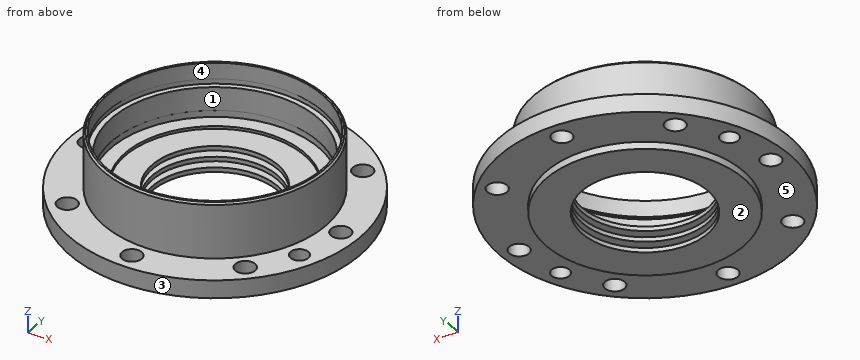
```python
from build123d import *

# Parameters (mm, degrees)
SKETCH_1_R               = 55
EXTRUDE_1_DEPTH          = 4
SKETCH_2_R               = 81
EXTRUDE_2_DEPTH          = 10
EXTRUDE_START            = 14
SKETCH_3_R               = 62
EXTRUDE_3_DEPTH          = 31
HOLE_WIZARD_1_D          = 11
PATTERN_CIRCULAR_1_COUNT = 8
HOLE_START               = 4
HOLE_WIZARD_2_OUTLINE_R  = 5
HOLE_WIZARD_2_DEPTH      = 10
CHAMFER_1_SIZE           = 1


# Read off the part's stored shape, not the designer's step: 孔2
with BuildPart() as part:
    # 草图1 → 凸台-拉伸1 (new body)
    with BuildSketch(Plane.XY):
        Circle(SKETCH_1_R)
    extrude(amount=EXTRUDE_1_DEPTH)

    # 草图2 → 凸台-拉伸2 (add)
    with BuildSketch(Plane.XY.offset(4)):
        Circle(SKETCH_2_R)
    extrude(amount=EXTRUDE_2_DEPTH)

    # 草图3 → 凸台-拉伸3 (add)
    with BuildSketch(Plane.XY.offset(EXTRUDE_START)):
        Circle(SKETCH_3_R)
    extrude(amount=EXTRUDE_3_DEPTH)

    # 草图4 → 切除-旋转1 (revolve, cut)
    with BuildSketch(Plane(origin=(0, 0, 0), x_dir=(0, 0, -1), z_dir=(1, 0, 0)), mode=Mode.PRIVATE) as cut_revolve_1_sk:
        Polygon((-45, 0), (-45, -60), (-36, -60), (-36, -60.5), (-33, -60.5), (-33, -57.5), (-20, -57.5), (-20, -58), (-16, -58), (-16, -50), (-14.5, -50), (-14.5, -35), (-12, -35), (-12, -40.6), (-8.5, -40.6), (-8.5, -35), (-6, -35), (-6, -40.6), (-2.5, -40.6), (-2.5, -35), (0, -35), (0, 0), align=None)
    revolve(cut_revolve_1_sk.sketch.rotate(Axis((0, 0, -13.139169211), (0, 0, 1)), 180), axis=Axis((0, 0, -13.139169211), (0, 0, 1)), mode=Mode.SUBTRACT)

    # 孔1 (through all)
    with Locations(Plane.XY.offset(14)):
        with Locations((-71, 0)):
            hole_wizard_1 = Hole(HOLE_WIZARD_1_D / 2)

    # 阵列(圆周)1: 孔1 ×8 about axis
    pattern_circular_1_axis = Axis((0, 0, 0), (0, 0, 1))
    for i in range(1, PATTERN_CIRCULAR_1_COUNT):
        add(hole_wizard_1.rotate(pattern_circular_1_axis, i * 360 / PATTERN_CIRCULAR_1_COUNT), mode=Mode.SUBTRACT)

    # 孔2 outline → 孔2 (cut)
    with BuildSketch(Plane.XY.offset(HOLE_START)):
        with Locations((-65.595446808, 27.170523698)):
            Circle(HOLE_WIZARD_2_OUTLINE_R)
        with Locations((65.595446808, -27.170523698)):
            Circle(HOLE_WIZARD_2_OUTLINE_R)
    extrude(amount=HOLE_WIZARD_2_DEPTH, mode=Mode.SUBTRACT)

    # 倒角1
    chamfer_1_edges = [part.edges().sort_by_distance(p)[0] for p in [
        (-62, 0, 45),
    ]]
    chamfer(chamfer_1_edges, length=CHAMFER_1_SIZE)


solid = part.part
```
Geometry: final body of the model. Coordinates: model frame, mm. Face numbers are marked on the shaded views. A direction names the side the tool comes from. Round coordinates to 2 decimals unless told otherwise and drop trailing zeros. Order: outer loops, then holes, each group sorted by start corner. A loop starts at its lowest first (then second) coordinate and runs counter-clockwise, first axis right, second up. Notation, with made-up numbers: (-14, 83) - (4, 83) arc R22 ccw to (4, 103) - close; hole circle Ø3 at (-28.75, 68.5). An arc over 180 degrees is marked (long way). Use CSV: the item, a comma, the result in double quotes. Start each with the question number.
Q1. Material intervals for line 1 along Z through (x, y) = (6.5, 38.5); line 2 along Y through (x, z) = (1, 3); line 3 along Z through (x, y) = (6, -43), sorted ascending. Write a range as from..to.
Q2. Access query for the marked faces 1 and 2. Directions: +Z, -Z, +X, -X, +Y, -Y. A direction counts if a zero-diameter tool reaches every point of the face in a straight line with its end or side. Return the directions, or none.
Q3. First-contact query: pin 1 (8 mm diameter, centred on y = 25, z = 13, fed in from -X); pin 2 (12 mm diameter, centred on y = -9.5, z = 33, fed in from +X); pin 3 (1.5 mm diameter, centred on y = 8.5, z = 15.5, fed in from -X); pin 4 (10 mm diameter, centred on x = 71, y = 0, fed in from +Z). Flat tips, straight axial feed; report the tip coordinate or a pass-through.
Q4. Section query C-C (z = 23.5). Return loops of the section in (x, y).
Q5. Section query B-B (y = 71). Return loops of the section in (x, z), and give its area (3 significant figures).
Q6. Section query A-A (x = 0). State how many separate pieces and enclosed holes the cut face has, and give its area (3 significant figures).
Q7. Mould query, pull axis Y, two halves, no side actions, for the marked faces 3, 4 and 5. Classes: +Y half, -Y half, draft (parallel to the pull), parting line (faces both ways), or undercut.
Result set:
1,line 1,"z = 0..2.5, 6..8.5, 12..14.5"
1,line 2,"y = -54.99..-40.59, 40.59..54.99"
1,line 3,"z = 0..14.5"
2,face 1,"+Z"
2,face 2,"-Z, +X, -X, +Y, -Y"
3,pin 1,"stops at x = -78.23"
3,pin 2,"stops at x = 61.9"
3,pin 3,"stops at x = -61.51"
3,pin 4,"passes through"
4,outline,"circle Ø124 at (0, 0); hole circle Ø115 at (0, 0)"
5,outline,"(-38.99, 4) - (-5.5, 4) - (-5.5, 14) - (-38.99, 14) - close; (5.5, 4) - (38.99, 4) - (38.99, 14) - (5.5, 14) - close"
5,area,"670 mm2"
6,separate pieces,"4"
6,enclosed holes,"0"
6,area,"1,040 mm2"
7,face 3,"parting line"
7,face 4,"undercut"
7,face 5,"draft"
